For this review, take the finished solid that the model builds, in its own axes (mm). Round coordinates to 2 decimals unless told otherwise and drop trailing zeros. Write each loop counter-clockwise with the first axis right and the second up, starting at its lowest first coordinate (ties: lowest second). Pieces come first, ordered by that corner, then holes. Notation, with made-up numbers: (18, 54) -> (34, 54) arc R10 cw to (34, 62) -> close; hole circle Ø3 at (79.5, 78.25). An arc over 180 degrees is marked (long way). Answer in a Markdown table with one row per item. Add a question column.
```python
from build123d import *

# Parameters (mm, degrees)
F0_W     = 290
F0_H     = 30
F1_DEPTH = 15
F3_D     = 5


# Not quite as in the source:
# - a feature names something its author has since deleted; it is built from what else it names


with BuildPart() as f1:
    # F0 (on Front) → F1 (new body, symmetric)
    with BuildSketch(Plane.XZ):
        Rectangle(F0_W, F0_H)
    extrude(amount=F1_DEPTH, both=True)

    # F3 (through all)
    with Locations(Plane.XZ.offset(15)):
        with Locations((-135, 5), (-135, -5), (-125, 5), (-125, -5), (125, 5), (125, -5), (135, 5), (135, -5)):
            Hole(F3_D / 2)


solid = f1.part
```
1. We need section B-B (y = 1.5). Count the separate pieces of the cut face and the enclosed holes in it, plus the area to 3 significant figures.
2. We need section C-C (z = -5). Write out the cut boundary in (x, y), plus the area to 3 significant figures.
3. For L1, parallel to Z at x = 135, y = -3.5; L2, parallel to X at y = -4, z = 6; L3, parallel to X at y = 12.5, z = -3, list the stretches that pass through material, from the lowest coordinate up. Write a range as [from, to].
4. The part is to be moulded in two halves that separate along X. For faces 1 (the cylindrical face through (122.615, 0.21, -4.249)), 2 (the cylindrical face through (-137.385, 0.21, 5.751)), 3 (the flat face through (-2, 0, 15)), 4 (the flat face through (145, 0, 0)), say which applies: pulls with the +X half, pulls with the -X half, needs draft (parallel to the pull), parting line crosses it, or undercut.
5. We need section A-A (x = 125). Write out the cut boundary in (y, z).
6. Clearance check with a flat-ended pin moving along its axis: pin 1 Ø3 at (x, z) = (135, 5) entering from -Y. State where the tip first meets the part, or that it passes through.
Response:
| question | item | result |
|---|---|---|
| 1 | separate pieces | 1 |
| 1 | enclosed holes | 8 |
| 1 | area | 8,540 mm2 |
| 2 | outline | (-145, -15) -> (-137.5, -15) -> (-137.5, 15) -> (-145, 15) -> close; (-132.5, -15) -> (-127.5, -15) -> (-127.5, 15) -> (-132.5, 15) -> close; (-122.5, -15) -> (122.5, -15) -> (122.5, 15) -> (-122.5, 15) -> close; (127.5, -15) -> (132.5, -15) -> (132.5, 15) -> (127.5, 15) -> close; (137.5, -15) -> (145, -15) -> (145, 15) -> (137.5, 15) -> close |
| 2 | area | 8,100 mm2 |
| 3 | L1 | [-15, -7.5], [-2.5, 2.5], [7.5, 15] |
| 3 | L2 | [-145, -137.29], [-132.71, -127.29], [-122.71, 122.71], [127.29, 132.71], [137.29, 145] |
| 3 | L3 | [-145, -136.5], [-133.5, -126.5], [-123.5, 123.5], [126.5, 133.5], [136.5, 145] |
| 4 | face 1 | undercut |
| 4 | face 2 | undercut |
| 4 | face 3 | needs draft |
| 4 | face 4 | pulls with the +X half |
| 5 | outline | (-15, -15) -> (15, -15) -> (15, -7.5) -> (-15, -7.5) -> close; (-15, -2.5) -> (15, -2.5) -> (15, 2.5) -> (-15, 2.5) -> close; (-15, 7.5) -> (15, 7.5) -> (15, 15) -> (-15, 15) -> close |
| 6 | pin 1 | through |
